Read the model definition and answer for the solid it produces. Units are mm, in the model's axes. Face numbers are marked on the shaded views. Give positions to 0.01 mm unless a question says otherwise; leave off trailing zeros. Order: outer loops, then holes, each group sorted by start corner. A loop starts at its lowest first (then second) coordinate and runs counter-clockwise, first axis right, second up. Notation, with made-up numbers: (-31, 35) - (-11, 35) arc R27 ccw to (-11, 68) - close; hole circle Ø2 at (31, 60.5). An arc over 180 degrees is marked (long way). Return JSON: item names as keys, results as strings.
```python
from build123d import *

# Parameters (mm, degrees)
SKETCH_1_W          = 4
SKETCH_1_H          = 4
EXTRUDE_1_DEPTH     = 30
SKETCH_4_W          = 8
SKETCH_4_H          = 2
CUT_EXTRUDE_1_DEPTH = 4
SKETCH_6_W          = 4
SKETCH_6_H          = 2
CUT_EXTRUDE_2_DEPTH = 2


with BuildPart() as part:
    # 草圖1 → 填料-伸長1 (new body)
    with BuildSketch(Plane.XY):
        Rectangle(SKETCH_1_W, SKETCH_1_H)
    extrude(amount=EXTRUDE_1_DEPTH)

    # 草圖4 → 除料-伸長1 (cut)
    with BuildSketch(Plane.ZY.offset(2)):
        with Locations((13, 1)):
            Rectangle(SKETCH_4_W, SKETCH_4_H)
    extrude(amount=-CUT_EXTRUDE_1_DEPTH, mode=Mode.SUBTRACT)

    # 草圖6 → 除料-伸長2 (cut)
    with BuildSketch(Plane.ZY.offset(2)):
        with Locations((13, -1)):
            Rectangle(SKETCH_6_W, SKETCH_6_H)
    extrude(amount=-CUT_EXTRUDE_2_DEPTH, mode=Mode.SUBTRACT)


solid = part.part
```
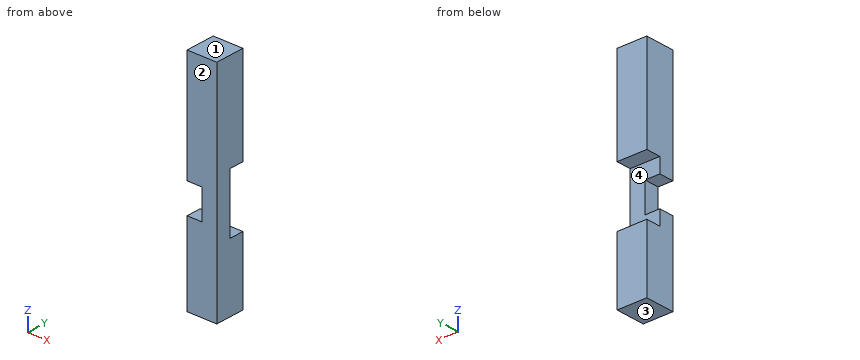
Q1. Determine the mould class of the marked faces 1, 2, 3 and 4 for opening direction Z: released by +Z, released by -Z, zero draft, split by the parting line, or undercut.
Values:
{"face 1": "released by +Z", "face 2": "zero draft", "face 3": "released by -Z", "face 4": "undercut"}
Q2. Given pin 1 (1 mm diameter, centred on y = -1.5, z = 12, fed in from -X); pin 2 (2 mm diameter, centred on x = 0.5, y = 0.5, fed in from -Z); pin 3 (1.2 mm diameter, centred on x = -0.5, z = 11.5, fed in from +Y), each flat-ended and moving along its own axis, determine where each tip first touches the part or whether it passes through.
Values:
{"pin 1": "stops at x = 0", "pin 2": "stops at z = 0", "pin 3": "stops at y = 0"}
Q3. Consider L1, parallel to Z at x = 1.65, y = 1.4; L2, parallel to Z at x = -0.25, y = -0.95; L3, parallel to X at y = -1.1, z = 11.5. Determine where each line is inside the solid, lowest interval first.
Values:
{"L1": "z = 0 to 9, 17 to 30", "L2": "z = 0 to 11, 15 to 30", "L3": "x = 0 to 2"}
Q4. A cutting plane is placed at B-B (x = -0.65). Write down the section's boundary in (y, z), and give its area (3 significant figures).
Values:
{"outline": "(-2, 0) - (2, 0) - (2, 9) - (0, 9) - (0, 11) - (-2, 11) - close; (-2, 15) - (0, 15) - (0, 17) - (2, 17) - (2, 30) - (-2, 30) - close", "area": "96.0 mm²"}
Q5. A cutting plane is placed at C-C (y = -1.25). Write down the section's boundary in (x, z).
Values:
{"outline": "(-2, 0) - (2, 0) - (2, 30) - (-2, 30) - (-2, 15) - (0, 15) - (0, 11) - (-2, 11) - close"}
Q6. A cutting plane is placed at A-A (y = 1.5). Write down the section's boundary in (x, z), and give its area (3 significant figures).
Values:
{"outline": "(-2, 0) - (2, 0) - (2, 9) - (-2, 9) - close; (-2, 17) - (2, 17) - (2, 30) - (-2, 30) - close", "area": "88.0 mm²"}
Q7. A cutting plane is placed at D-D (x = 0.9). Write down the section's boundary in (y, z), and give its area (3 significant figures).
Values:
{"outline": "(-2, 0) - (2, 0) - (2, 9) - (0, 9) - (0, 17) - (2, 17) - (2, 30) - (-2, 30) - close", "area": "104 mm²"}
